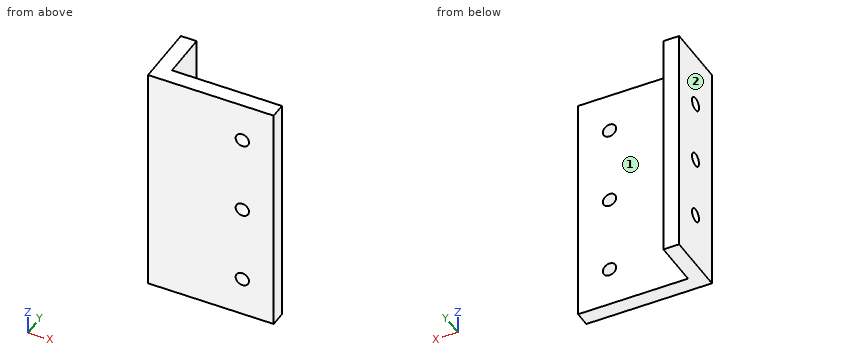
from build123d import *

# Parameters (mm, degrees)
EXTRUDE_1_DEPTH                   = 150
HOLE_WIZARD_8_5_8_5_1_D           = 8.5
HOLE_WIZARD_8_5_8_5_1_ON_FACE_2_D = 8.5


with BuildPart() as part:
    # 草图1 → 凸台-拉伸1 (new body)
    with BuildSketch(Plane.XY):
        Polygon((0, 40), (0, 0), (80, 0), (80, 10), (10, 10), (10, 40), align=None)
    extrude(amount=EXTRUDE_1_DEPTH)

    # Ø8.5 (8.5) 直径孔1 (through all)
    with Locations(Plane(origin=(10, 20, 115), x_dir=(0, 0, 1), z_dir=(1, 0, 0))):
        with Locations((0, 0), (-80, 0), (-40, 0)):
            Hole(HOLE_WIZARD_8_5_8_5_1_D / 2)

    # Ø8.5 (8.5) 直径孔1 on face 2 (through all)
    with Locations(Plane(origin=(60, 10, 125), x_dir=(0, 0, 1), z_dir=(0, 1, 0))):
        with Locations((0, 0), (-100, 0), (-50, 0)):
            Hole(HOLE_WIZARD_8_5_8_5_1_ON_FACE_2_D / 2)


solid = part.part
The listing builds one solid part. Answer for the finished solid, in the listing's coordinates (mm). Face numbers are marked on the shaded views. A direction names the side the tool comes from. Round coordinates to 2 decimals unless told otherwise and drop trailing zeros. Write each loop counter-clockwise with the first axis right and the second up, starting at its lowest first coordinate (ties: lowest second). Pieces come first, ordered by that corner, then holes. Notation, with made-up numbers: M 10,-26 L 23,-26 A19 ccw 23,11 Z; hole C 18.5,72.5 d1. An arc over 180 degrees is marked long. Write each question's results on one line, items separated by ' | '. Start each with the question number.
(1) For the marked faces 1 and 2, determine the directions among +Z, -Z, +X, -X, +Y, -Y from which every point of the face is accessible in a straight line to the end or side of a thin tool.
(2) The part is cut by section D-D, the plane z = 125. Write down the section's boundary in (x, y).
(3) The part is cut by section A-A, the plane y = 20. Write down the section's boundary in (x, z), and give its area (4 significant figures).
(4) Each of these flat-tipped pins is pushed along its axis until it touches: P1, Ø1.5, axis at x = 56, z = 129.5, coming from the +Y side; P2, Ø13.5, axis at y = 20, z = 75, coming from the +X side; P3, Ø5, axis at x = 60, z = 125, coming from the -Y side. Where does it stop, or does it pass through?
(5) The part is cut by section C-C, the plane z = 75. Write down the section's boundary in (x, y), and give its area (3 significant figures).
(6) Find the intervals of material crossed by line 1 (Z direction, x = 3, y = 20); line 2 (X direction, y = 34, z = 44), in increasing order.
(7) The part is cut by section B-B, the plane x = 60. Write down the section's boundary in (y, z).
Worked answers:
1) face 1: +Z, -Z, +X, +Y | face 2: +Z, -Z, -X, +Y, -Y
2) outline: M 0,0 L 55.75,0 L 55.75,10 L 10,10 L 10,40 L 0,40 Z; M 64.25,0 L 80,0 L 80,10 L 64.25,10 Z
3) outline: M 0,0 L 10,0 L 10,30.75 L 0,30.75 Z; M 0,39.25 L 10,39.25 L 10,70.75 L 0,70.75 Z; M 0,79.25 L 10,79.25 L 10,110.75 L 0,110.75 Z; M 0,119.25 L 10,119.25 L 10,150 L 0,150 Z | area: 1,245 mm²
4) P1: stops at y = 10 | P2: stops at x = 10 | P3: passes through
5) outline: M 0,0 L 55.75,0 L 55.75,10 L 10,10 L 10,15.75 L 0,15.75 Z; M 0,24.25 L 10,24.25 L 10,40 L 0,40 Z; M 64.25,0 L 80,0 L 80,10 L 64.25,10 Z | area: 930 mm²
6) line 1: z = 0 to 30.75, 39.25 to 70.75, 79.25 to 110.75, 119.25 to 150 | line 2: x = 0 to 10
7) outline: M 0,0 L 10,0 L 10,20.75 L 0,20.75 Z; M 0,29.25 L 10,29.25 L 10,70.75 L 0,70.75 Z; M 0,79.25 L 10,79.25 L 10,120.75 L 0,120.75 Z; M 0,129.25 L 10,129.25 L 10,150 L 0,150 Z
